Check sheet for the modelled part. Datum: model origin and axes. Units: mm. Give positions to 0.01 mm unless a question says otherwise; leave off trailing zeros. Order: outer loops, then holes, each group sorted by start corner. A loop starts at its lowest first (then second) coordinate and runs counter-clockwise, first axis right, second up.
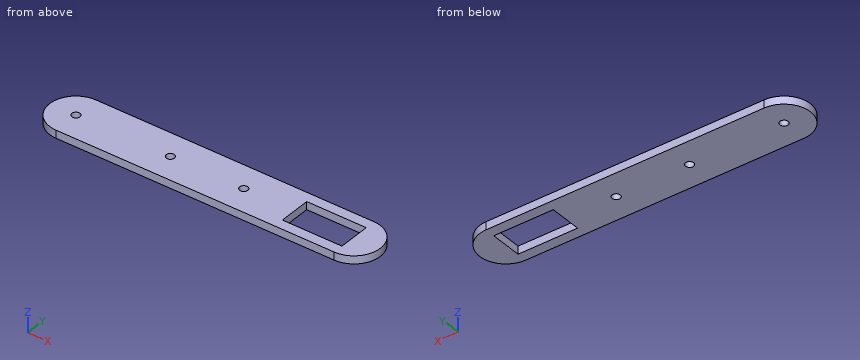
```python
from build123d import *

# Parameters (mm, degrees)
BOSS_EXTRUDE1_DEPTH = 3
SKETCH3_R           = 1.55
CUT_EXTRUDE2_DEPTH  = 3
SKETCH4_R           = 1.55
CUT_EXTRUDE4_DEPTH  = 3
SKETCH5_R           = 1.55
CUT_EXTRUDE6_DEPTH  = 3
SKETCH6_W           = 22.7
SKETCH6_H           = 12.2
CUT_EXTRUDE7_DEPTH  = 3


with BuildPart() as part:
    # Sketch1 → Boss-Extrude1 (new body)
    with BuildSketch(Plane.XY):
        with BuildLine():
            Line((-58.058617241, 24.191090517), (47.991382759, 24.191090517))
            ThreePointArc((47.991382759, 24.191090517), (57.991382759, 14.191090517), (47.991382759, 4.191090517))
            Line((47.991382759, 4.191090517), (-58.058617241, 4.191090517))
            ThreePointArc((-58.058617241, 4.191090517), (-68.058617241, 14.191090517), (-58.058617241, 24.191090517))
        make_face()
    extrude(amount=BOSS_EXTRUDE1_DEPTH)

    # Sketch3 → Cut-Extrude2 (cut)
    with BuildSketch(Plane.XY.offset(3)):
        with Locations((-58.058617241, 14.191090517)):
            Circle(SKETCH3_R)
    extrude(amount=-CUT_EXTRUDE2_DEPTH, mode=Mode.SUBTRACT)

    # Sketch4 → Cut-Extrude4 (cut)
    with BuildSketch(Plane(origin=(9.979459273, 1.433252018, 3), x_dir=(1, 0, 0), z_dir=(0, 0, 1))):
        with Locations((-4.038076514, 12.757838499)):
            Circle(SKETCH4_R)
    extrude(amount=-CUT_EXTRUDE4_DEPTH, mode=Mode.SUBTRACT)

    # Sketch5 → Cut-Extrude6 (cut)
    with BuildSketch(Plane(origin=(-9.979459273, 1.433252018, 0), x_dir=(-1, 0, 0), z_dir=(0, 0, -1))):
        with Locations((12.079157968, 12.757838499)):
            Circle(SKETCH5_R)
    extrude(amount=-CUT_EXTRUDE6_DEPTH, mode=Mode.SUBTRACT)

    # Sketch6 → Cut-Extrude7 (cut)
    with BuildSketch(Plane.XY.offset(3)):
        with Locations((36.641382759, 14.191090517)):
            Rectangle(SKETCH6_W, SKETCH6_H)
    extrude(amount=-CUT_EXTRUDE7_DEPTH, mode=Mode.SUBTRACT)


solid = part.part
```
(1) Cross-section at C-C on z = 1.5. Enter the section's corners in (x, y).
Response values:
outline: (-58.06, 4.19) - (47.99, 4.19) arc R10 ccw to (47.99, 24.19) - (-58.06, 24.19) arc R10 ccw to start; hole circle Ø3.1 at (-58.06, 14.19); hole circle Ø3.1 at (-22.06, 14.19); hole circle Ø3.1 at (5.94, 14.19); hole (25.29, 8.09) - (47.99, 8.09) - (47.99, 20.29) - (25.29, 20.29) - close
(2) Cross-section at B-B on y = 19.25. Enter the section's corners in (x, z), then the cut area to 3 significant figures.
Response values:
outline: (-66.68, 0) - (25.29, 0) - (25.29, 3) - (-66.68, 3) - close; (47.99, 0) - (56.62, 0) - (56.62, 3) - (47.99, 3) - close
area: 302 mm2
(3) Cross-section at A-A on x = 44. Enter the section's corners in (y, z), then the cut area to 3 significant figures.
Response values:
outline: (4.19, 0) - (8.09, 0) - (8.09, 3) - (4.19, 3) - close; (20.29, 0) - (24.19, 0) - (24.19, 3) - (20.29, 3) - close
area: 23.4 mm2
(4) Material ranges on L1, parallel to Y at x = 46, z = 1.35; L2, parallel to X at y = 16.75, z = 1.5; L3, parallel to X at y = 11, z = 1.1, recorded low to high.
Response values:
L1: y = 4.19 to 8.09, 20.29 to 24.19
L2: x = -67.73 to 25.29, 47.99 to 57.66
L3: x = -67.54 to 25.29, 47.99 to 57.47
